Work out the finished part from the listing and answer in its coordinate system (mm). Face numbers are marked on the shaded views. A direction names the side the tool comes from. Round coordinates to 2 decimals unless told otherwise and drop trailing zeros. Order: outer loops, then holes, each group sorted by start corner. A loop starts at its lowest first (then second) coordinate and runs counter-clockwise, first axis right, second up. Notation, with made-up numbers: (-38.75, -20.5) - (-26.75, -20.5) arc R16 cw to (-26.75, -16.5) - close; hole circle Ø3 at (66.25, 69). An arc over 180 degrees is marked (long way). Use one line per item in the form item = value. Start each with the question number.
Q1. Which of the six approach directions +Z, -Z, +X, -X, +Y, -Y give full straight-line access (tool end or side, diameter ignored) to the marked faces 5 and 6?
Q2. For a pull along Y with two mould halves and no side action, classify the marked faces 1, 2, 3 and 4 as +Y half, -Y half, draft (parallel to the pull), parting line (faces both ways), or undercut.
Q3. Find the intervals of material crossed by line 1 (X direction, y = 13, z = -4.5); line 2 (Z direction, x = 15.5, y = 3); line 3 (X direction, y = 6.75, z = -17), in increasing order. Write a range as [from, to].
Q4. The part is cut by section D-D on z = -16. Determine the outline of the cut face in (x, y), plus the area to 3 significant figures.
Q5. The part is cut by section C-C on x = 20.5. Determine the outline of the cut face in (y, z), plus the area to 3 significant figures.
Q6. The part is cut by section B-B on z = -5. Determine the outline of the cut face in (x, y), plus the area to 3 significant figures.
Q7. The part is cut by section A-A on y = 13.75. Determine the outline of the cut face in (x, z), plus the area to 3 significant figures.
from build123d import *

# Parameters (mm, degrees)
BOSS_EXTRUDE1_DEPTH = 20.1168
SKETCH2_R           = 6.75
BOSS_EXTRUDE2_DEPTH = 2
SKETCH3_R           = 2.945
BOSS_EXTRUDE3_DEPTH = 4


with BuildPart() as part:
    # Sketch1 → Boss-Extrude1 (new body)
    with BuildSketch(Plane(origin=(0, 0, 0), x_dir=(1, 0, 0), z_dir=(0, 1, 0))):
        Polygon((19.9009, -12.278622803), (15.0749, -20.6375), (-19.9009, -20.6375), (-19.9009, 20.6375), (19.9009, 20.6375), align=None)
    extrude(amount=BOSS_EXTRUDE1_DEPTH)

    # Sketch2 → Boss-Extrude2 (add)
    with BuildSketch(Plane(origin=(19.9009, 0, 0), x_dir=(0, 0, -1), z_dir=(1, 0, 0))):
        with Locations(Location((10.4375, 10.0584, 0), (0, 0, 180))):
            Circle(SKETCH2_R)
    extrude(amount=BOSS_EXTRUDE2_DEPTH)

    # Sketch3 → Boss-Extrude3 (add)
    with BuildSketch(Plane(origin=(21.9009, 0, 0), x_dir=(0, 0, -1), z_dir=(1, 0, 0))):
        with Locations((10.4375, 10.0584)):
            Circle(SKETCH3_R)
    extrude(amount=BOSS_EXTRUDE3_DEPTH)


solid = part.part
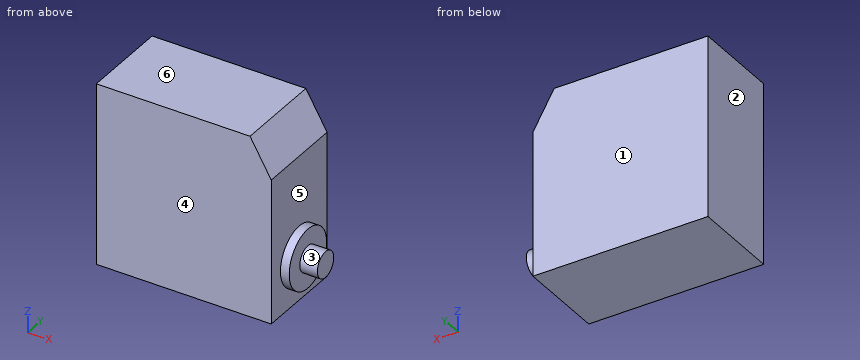
Found:
q1.face_5 = +X
q1.face_6 = +Z, +X, -X, +Y, -Y
q2.face_1 = +Y half
q2.face_2 = draft
q2.face_3 = parting line
q2.face_4 = -Y half
q3.line_1 = [-19.9, 21.9]
q3.line_2 = [-20.64, 19.9]
q3.line_3 = [-19.9, 19.9]
q4.outline = (-19.9, 0) - (19.9, 0) - (19.9, 6.23) - (21.9, 6.23) - (21.9, 13.88) - (19.9, 13.88) - (19.9, 20.12) - (-19.9, 20.12) - close
q4.area = 816 mm²
q5.outline = circle Ø13.5 at (10.06, -10.44)
q5.area = 143 mm²
q6.outline = (-19.9, 0) - (19.9, 0) - (19.9, 6.06) - (21.9, 6.06) - (21.9, 14.06) - (19.9, 14.06) - (19.9, 20.12) - (-19.9, 20.12) - close
q6.area = 817 mm²
q7.outline = (-19.9, -20.64) - (19.9, -20.64) - (19.9, -16.09) - (21.9, -16.09) - (21.9, -4.79) - (19.9, -4.79) - (19.9, 12.28) - (15.07, 20.64) - (-19.9, 20.64) - close
q7.area = 1,650 mm²
